Geometry: final body of the model. Coordinates: model frame, mm. Face numbers are marked on the shaded views. Give positions to 0.01 mm unless a question says otherwise; leave off trailing zeros. Write each loop counter-clockwise with the first axis right and the second up, starting at its lowest first coordinate (ties: lowest second). Pieces come first, ordered by that corner, then holes. Notation, with made-up numbers: M 40,86.25 L 94,86.25 A25 cw 94,121.25 Z; hole C 25.25,21.25 d10. An arc over 180 degrees is marked long. Use one line per item in the form item = value. Start each with the question number.
Item 1: Section query B-B on z = 6. Return loops of the section in (x, y), then the cut area to 3 significant figures.
Item 2: Pull-direction query (X, two-part tool) for the marked faces 1, 2 and 3; classes: released by +X, released by -X, zero draft, split by the parting line, or undercut.
Item 3: Section query D-D on y = 6. Return loops of the section in (x, z), then the cut area to 3 significant figures.
Item 4: Material intervals for line 1 along X through (y, z) = (4.4, 0); line 2 along Y through (x, z) = (20.5, 5.5); line 3 along Z through (x, y) = (0, 6), sorted ascending. Write a range as from..to.
Item 5: Section query C-C on x = -13. Return loops of the section in (y, z), then the cut area to 3 significant figures.
Item 6: Section query A-A on z = 0. Return loops of the section in (x, y).
Item 7: Contact query for a flat-ended pin moving along its axis: P1, Ø11.5, axis at x = 0, z = 0, coming from the +Y side. Output: stop coordinate, or through.
Autodesk Inventor part; units mm, degrees
ref_plane "YZ Plane" through (0, 0, 0) normal (1, 0, 0) x (0, 1, 0)
ref_plane "XZ Plane" through (0, 0, 0) normal (0, 1, 0) x (-1, 0, 0)
ref_plane "XY Plane" through (0, 0, 0) normal (0, 0, 1) x (1, 0, 0)
sketch "Эскиз4" plane through (0, 0, 0) normal (0, 1, 0) x (-1, 0, 0)
  line L0 (30, 20) -> (-30, 20)
  line L1 (-30, 20) -> (-30, -20)
  line L2 (-30, -20) -> (30, -20)
  line L3 (30, -20) -> (30, 20)
  point P0 (0, 0)
  dimension "d16" = 40
  dimension "d17" = 20
  dimension "d18" = 60
  dimension "d19" = 30
extrude "Выдавливание4" add sketch "Эскиз4" along normal mid plane 15
sketch "Эскиз6" plane through (30, -7.5, -20) normal (1, 0, 0) x (0, 0, -1)
  line L0 (-12.5, 5) -> (-27.5, 5)
  line L1 (-27.5, 5) -> (-27.5, 10)
  line L2 (-27.5, 10) -> (-12.5, 10)
  line L3 (-12.5, 10) -> (-12.5, 5)
  point P0 (-20, 7.5)
  dimension "d25" = 5
  dimension "d26" = 15
  dimension "d27" = 7.5
  dimension "d28" = 2.5
extrude "Выдавливание5" cut sketch "Эскиз6" against normal through all
sketch "Эскиз7" plane through (0, 7.5, 0) normal (0, 1, 0) x (1, 0, 0)
  point P0 (0, 0)
  point P1 (0, 0)
hole "Отверстие2" at (0, 7.5, 0) direction (0, -1, 0) diameter 10 depth 5
properties part number "Каменъ"
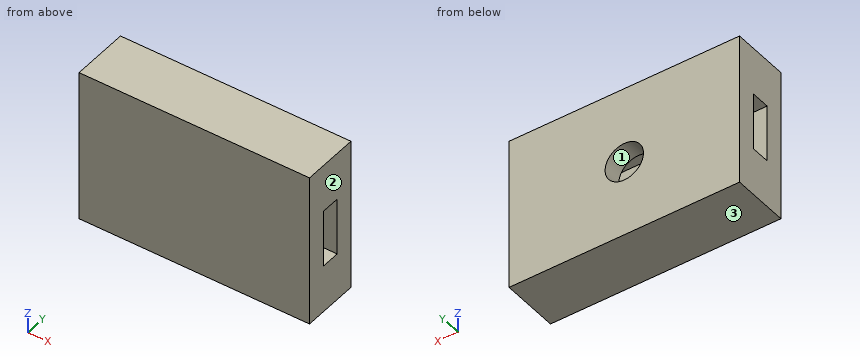
Answer sheet:
q1.outline = M -30,-7.5 L 30,-7.5 L 30,-2.5 L -30,-2.5 Z; M -30,2.5 L 30,2.5 L 30,7.5 L -30,7.5 Z
q1.area = 600 mm2
q2.face_1 = undercut
q2.face_2 = released by +X
q2.face_3 = zero draft
q3.outline = M -30,-20 L 30,-20 L 30,20 L -30,20 Z; hole C 0,0 d10
q3.area = 2,320 mm2
q4.line_1 = -30..-5, 5..30
q4.line_2 = -7.5..-2.5, 2.5..7.5
q4.line_3 = -20..-5, 5..20
q5.outline = M -7.5,-20 L 7.5,-20 L 7.5,20 L -7.5,20 Z; hole M -2.5,-7.5 L 2.5,-7.5 L 2.5,7.5 L -2.5,7.5 Z
q5.area = 525 mm2
q6.outline = M -30,-7.5 L 30,-7.5 L 30,-2.5 L -30,-2.5 Z; M -30,2.5 L -5,2.5 L -5,7.5 L -30,7.5 Z; M 5,2.5 L 30,2.5 L 30,7.5 L 5,7.5 Z
q7.P1 = 7.5
